Geometry check sheet. Reference: drawing and pictorial views, mm from the part's lowest x, y, z. A direction names the side the tool comes from. Give positions to 0.01 mm unless a question says otherwise; leave off trailing zeros. Order: outer loops, then holes, each group sorted by start corner. A loop starts at its lowest first (then second) coordinate and runs counter-clockwise, first axis right, second up.
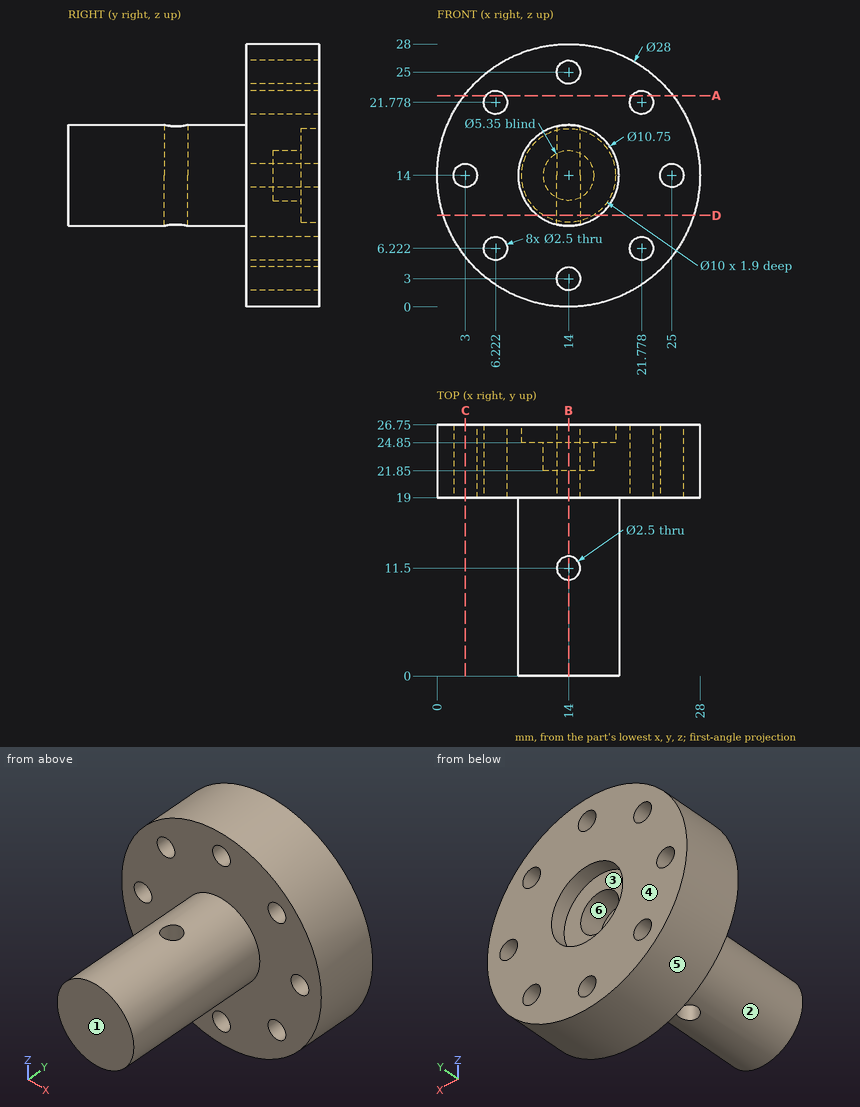
1) Depth check by flat-ended pin: pin 1 Ø1.5 at (x, z) = (14, 25) entering from -Y; pin 2 Ø12 at (x, z) = (5.5, 18.5) entering from -Y; pin 3 Ø9 at (x, z) = (14, 14) entering from +Y; pin 4 Ø1 at (x, z) = (12, 14) entering from +Y. Enter the tip coordinate at first touch or a pass-through.
Recorded:
pin 1: passes through
pin 2: stops at y = 0
pin 3: stops at y = 24.85
pin 4: stops at y = 21.85
2) Section check A-A, the plane z = 22.5. Record the cut outline in (x, y).
Recorded:
outline: (2.88, 19) - (5.2, 19) - (5.2, 26.75) - (2.88, 26.75) - close; (7.24, 19) - (20.76, 19) - (20.76, 26.75) - (7.24, 26.75) - close; (22.8, 19) - (25.12, 19) - (25.12, 26.75) - (22.8, 26.75) - close
3) Material ranges on L1, parallel to Z at x = 14, y = 24 (3 decimals); L2, parallel to Y at x = 9.25, z = 22.75, recorded low to high.
Recorded:
L1: z = 0 to 1.75, 4.25 to 11.325, 16.675 to 23.75, 26.25 to 28
L2: y = 19 to 26.75
4) Section check B-B, the plane x = 14. Record the cut outline in (y, z) (3 decimals).
Recorded:
outline: (0, 8.625) - (10.25, 8.625) - (10.25, 19.375) - (0, 19.375) - close; (12.75, 8.625) - (19, 8.625) - (19, 4.25) - (26.75, 4.25) - (26.75, 9) - (24.85, 9) - (24.85, 11.325) - (21.85, 11.325) - (21.85, 16.675) - (24.85, 16.675) - (24.85, 19) - (26.75, 19) - (26.75, 23.75) - (19, 23.75) - (19, 19.375) - (12.75, 19.375) - close; (19, 0) - (26.75, 0) - (26.75, 1.75) - (19, 1.75) - close; (19, 26.25) - (26.75, 26.25) - (26.75, 28) - (19, 28) - close
5) Section check D-D, the plane z = 9.75. Record the cut outline in (x, y).
Recorded:
outline: (0.66, 19) - (10.71, 19) - (10.71, 0) - (17.29, 0) - (17.29, 19) - (27.34, 19) - (27.34, 26.75) - (16.63, 26.75) - (16.63, 24.85) - (11.37, 24.85) - (11.37, 26.75) - (0.66, 26.75) - close; hole circle Ø2.5 at (14, 11.5)
6) Set-up check for the marked faces 1, 2 and 3: record each of +Z, -Z, +X, -X, +Y, -Y from which the full face is reachable in a straight line by a thin tool's end or side.
Recorded:
face 1: +Z, -Z, +X, -X, -Y
face 2: -Y
face 3: +Y
7) Section check C-C, the plane x = 3. Record the cut outline in (y, z), then the cut area to 3 significant figures.
Recorded:
outline: (19, 5.34) - (26.75, 5.34) - (26.75, 12.75) - (19, 12.75) - close; (19, 15.25) - (26.75, 15.25) - (26.75, 22.66) - (19, 22.66) - close
area: 115 mm2
8) Draft check along X on the marked faces 4, 5 and 6. Enter one of: +X half, -X half, draft (parallel to the pull), parting line (faces both ways), or undercut.
Recorded:
face 4: draft
face 5: parting line
face 6: undercut
